Geometry: see drawing. Coordinates: mm, zero at the bounding-box minimum. A direction names the side the tool comes from. Round coordinates to 2 decimals unless told otherwise and drop trailing zeros. Write each loop counter-clockwise with the first axis right and the second up, starting at its lowest first coordinate (ties: lowest second). Pieces come first, ordered by that corner, then holes.
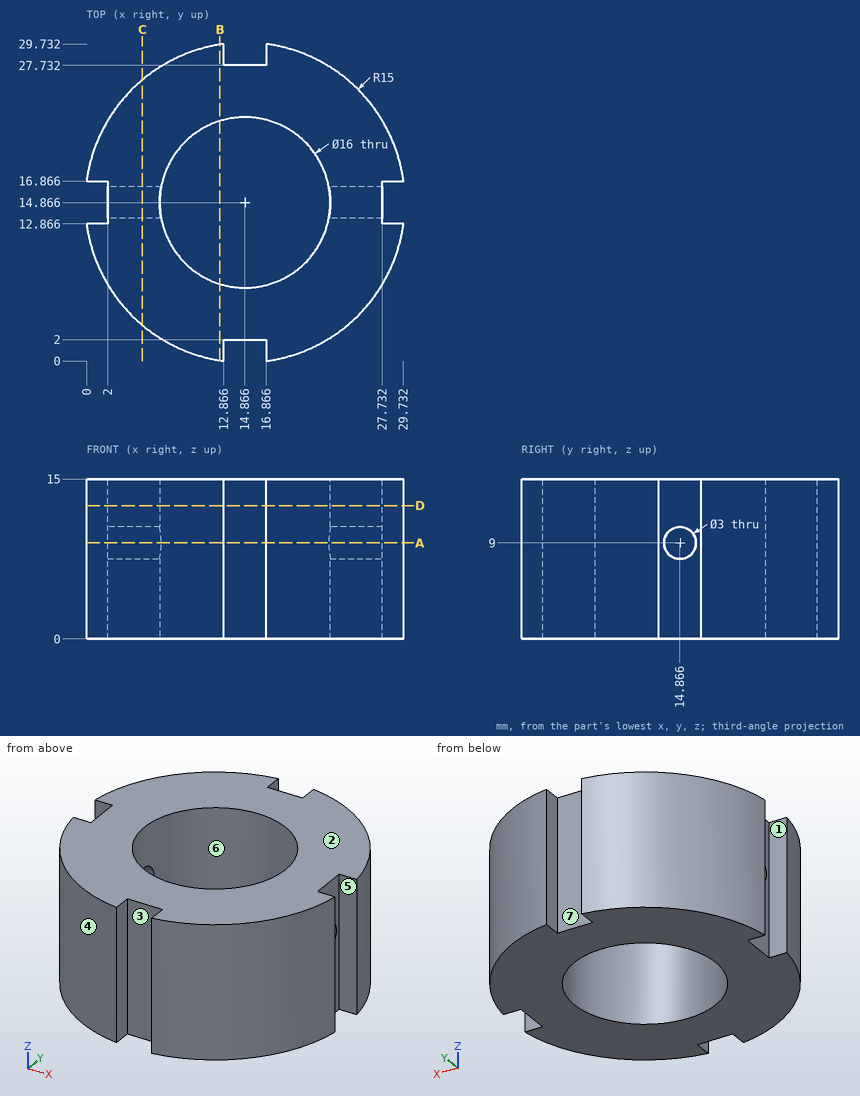
1) Section query D-D on z = 12.5. Return the cut outline in (x, y).
Taken from the geometry:
outline: (0, 12.87) arc R15 ccw to (12.87, 0) - (12.87, 2) - (16.87, 2) - (16.87, 0) arc R15 ccw to (29.73, 12.87) - (27.73, 12.87) - (27.73, 16.87) - (29.73, 16.87) arc R15 ccw to (16.87, 29.73) - (16.87, 27.73) - (12.87, 27.73) - (12.87, 29.73) arc R15 ccw to (0, 16.87) - (2, 16.87) - (2, 12.87) - close; hole circle Ø16 at (14.87, 14.87)
2) Section query B-B on x = 12.5. Return the cut outline in (y, z), then the cut area to 3 significant figures.
Taken from the geometry:
outline: (0.05, 0) - (7.22, 0) - (7.22, 15) - (0.05, 15) - close; (22.51, 0) - (29.68, 0) - (29.68, 15) - (22.51, 15) - close
area: 215 mm2
3) Section query A-A on z = 9. Return the cut outline in (x, y).
Taken from the geometry:
outline: (0, 12.87) arc R15 ccw to (12.87, 0) - (12.87, 2) - (16.87, 2) - (16.87, 0) arc R15 ccw to (29.73, 12.87) - (27.73, 12.87) - (27.73, 13.37) - (22.72, 13.37) arc R8 cw to (7.01, 13.37) - (2, 13.37) - (2, 12.87) - close; (0, 16.87) - (2, 16.87) - (2, 16.37) - (7.01, 16.37) arc R8 cw to (22.72, 16.37) - (27.73, 16.37) - (27.73, 16.87) - (29.73, 16.87) arc R15 ccw to (16.87, 29.73) - (16.87, 27.73) - (12.87, 27.73) - (12.87, 29.73) arc R15 ccw to start
4) Section query C-C on x = 5.25. Return the cut outline in (y, z).
Taken from the geometry:
outline: (3.35, 0) - (26.38, 0) - (26.38, 15) - (3.35, 15) - close; hole circle Ø3 at (14.87, 9)
5) Pull-direction query (Y, two-part tool) for the marked faces 4, 5, 6 and 7; classes: released by +Y, released by -Y, zero draft, split by the parting line, or undercut.
Taken from the geometry:
face 4: released by -Y
face 5: undercut
face 6: undercut
face 7: released by +Y
6) Material intervals for line 1 (X direction, y = 14.25, z = 3.5); line 2 (X direction, y = 7.5, z = 5.5) (1 decimal); line 3 (Y direction, x = 17.75, z = 14), sorted ascending.
Taken from the geometry:
line 1: x = 2 to 6.89, 22.84 to 27.73
line 2: x = 1.8 to 11.7, 18 to 27.9
line 3: y = 0.15 to 7.4, 22.33 to 29.59
7) Contact query for flat-ended pins moving along their axis: P1, Ø1.6, axis at y = 28.5, z = 9.5, coming from the -X side; P2, Ø6, axis at y = 24, z = 11.5, coming from the -X side; P3, Ø1.6, axis at y = 1.5, z = 10.5, coming from the +X side. Output: stop coordinate, or through.
Taken from the geometry:
P1: stops at x = 7.1
P2: stops at x = 1.18
P3: stops at x = 23.06
8) Reachability of the marked faces 1, 2 and 3 from +Z, -Z, +X, -X, +Y, -Y: full face, straight path, thin tool, end or side. Return the list, or none.
Taken from the geometry:
face 1: +Z, -Z, -X
face 2: +Z, +X, -X, +Y, -Y
face 3: +Z, -Z, -Y
